from build123d import *

# Parameters (mm, degrees)
F1_DEPTH = 3.81
F2_R     = 8.89
F3_DEPTH = 2.54
F4_R     = 7.493
F5_DEPTH = 3.175
F6_R     = 0.4911819864


with BuildPart() as f1:
    # F0 (on Front) → F1 (new body)
    with BuildSketch(Plane.XZ):
        with BuildLine():
            ThreePointArc((8.8754738465, -0.508), (8.8863677196, -0.2541038219), (8.89, 0))
            ThreePointArc((8.89, 0), (7.6804215502, 4.4769660275), (4.3808380628, 7.7356549734))
            add(Edge.make_bspline(
                [(2.7757389763, 8.4455534535), (3.2888417453, 8.2703062234), (3.8159102337, 8.0198976132), (4.3808380628, 7.7356549734)],
                knots=[0.1783179795, 0.1783179795, 0.1783179795, 0.1783179795, 0.2655314771, 0.2655314771, 0.2655314771, 0.2655314771], degree=3))
            ThreePointArc((2.7757389763, 8.4455534535), (2.4438853282, 8.5474864435), (2.1083049646, 8.6363852494))
            add(Edge.make_bspline(
                [(0, 8.89), (0.577506035, 8.8570186599), (1.3119112895, 8.8227589155), (2.1083049646, 8.6363852494)],
                knots=[0, 0, 0, 0, 0.1399319156, 0.1399319156, 0.1399319156, 0.1399319156], degree=3))
            add(Edge.make_bspline(
                [(0, 8.89), (-0.577506035, 8.8570186599), (-1.3119112895, 8.8227589155), (-2.1083049646, 8.6363852494)],
                knots=[0, 0, 0, 0, 0.1399319156, 0.1399319156, 0.1399319156, 0.1399319156], degree=3))
            ThreePointArc((-2.1083049646, 8.6363852494), (-2.4438853282, 8.5474864435), (-2.7757389763, 8.4455534535))
            add(Edge.make_bspline(
                [(-2.7757389763, 8.4455534535), (-3.2888417453, 8.2703062234), (-3.8159102337, 8.0198976132), (-4.3808380628, 7.7356549734)],
                knots=[0.1783179795, 0.1783179795, 0.1783179795, 0.1783179795, 0.2655314771, 0.2655314771, 0.2655314771, 0.2655314771], degree=3))
            ThreePointArc((-4.3808380628, 7.7356549734), (-7.8052490793, 4.255606515), (-8.8754738465, -0.508))
            Line((-8.8754738465, -0.508), (-5.2194662387, -0.508))
            Line((-5.2194662387, -0.508), (-5.7473639175, 0.0198976788))
            Line((-5.7473639175, 0.0198976788), (0, 5.7672615963))
            Line((0, 5.7672615963), (5.7473639175, 0.0198976788))
            Line((5.7473639175, 0.0198976788), (5.2194662387, -0.508))
            Line((5.2194662387, -0.508), (8.8754738465, -0.508))
        make_face()
        with BuildLine():
            ThreePointArc((4.3808380628, 7.7356549734), (7.6804215502, 4.4769660275), (8.89, 0))
            ThreePointArc((8.89, 0), (8.8863677196, -0.2541038219), (8.8754738465, -0.508))
            Line((8.8754738465, -0.508), (20.32, -0.508))
            add(Edge.make_bspline(
                [(4.3808380628, 7.7356549734), (5.5525412949, 7.1461141461), (9.398567587, 5.0276978273), (19.2176653381, 4.6545545686), (20.0494547253, 0.2736910266), (20.32, -0.508)],
                knots=[0.2655314771, 0.2655314771, 0.2655314771, 0.2655314771, 0.4464188962, 0.7868227895, 1, 1, 1, 1], degree=3))
        make_face()
        with BuildLine():
            ThreePointArc((-8.8754738465, -0.508), (0, -8.89), (8.8754738465, -0.508))
            Line((8.8754738465, -0.508), (5.2194662387, -0.508))
            Line((5.2194662387, -0.508), (0, -5.7274662387))
            Line((0, -5.7274662387), (-5.2194662387, -0.508))
            Line((-5.2194662387, -0.508), (-8.8754738465, -0.508))
        make_face()
        with BuildLine():
            Line((-20.32, -0.508), (-8.8754738465, -0.508))
            ThreePointArc((-8.8754738465, -0.508), (-7.8052490793, 4.255606515), (-4.3808380628, 7.7356549734))
            add(Edge.make_bspline(
                [(-4.3808380628, 7.7356549734), (-5.5525412949, 7.1461141461), (-9.398567587, 5.0276978273), (-19.2176653381, 4.6545545686), (-20.0494547253, 0.2736910266), (-20.32, -0.508)],
                knots=[0.2655314771, 0.2655314771, 0.2655314771, 0.2655314771, 0.4464188962, 0.7868227895, 1, 1, 1, 1], degree=3))
        make_face()
    extrude(amount=F1_DEPTH)

    # F2 (on face) → F3 (join)
    with BuildSketch(Plane.XZ.offset(3.81)):
        Circle(F2_R)
        Polygon((-5.7473639175, 0.0198976788), (0, 5.7672615963), (5.7473639175, 0.0198976788), (0, -5.7274662387), align=None, mode=Mode.SUBTRACT)
    extrude(amount=F3_DEPTH)

    # F4 (on face) → F5 (join)
    with BuildSketch(Plane.XZ.offset(6.35)):
        Circle(F4_R)
        Polygon((0, -5.7274662387), (-5.7473639175, 0.0198976788), (0, 5.7672615963), (5.7473639175, 0.0198976788), align=None, mode=Mode.SUBTRACT)
    extrude(amount=F5_DEPTH)

    # F6
    f6_edges = [f1.edges().sort_by_distance(p)[0] for p in [
        (20.32, -1.905, -0.508),
        (-20.32, -1.905, -0.508),
    ]]
    fillet(f6_edges, radius=F6_R)


solid = f1.part
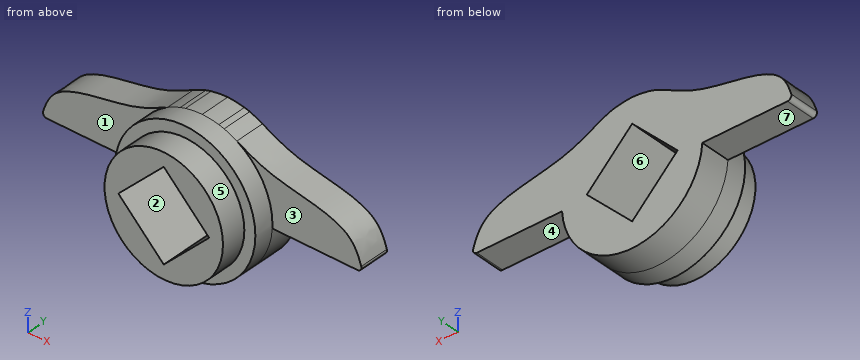
Could you check a few things on this model? Use its own coordinates, in mm. Face numbers are marked on the shaded views. A direction names the side the tool comes from. Round coordinates to 2 decimals unless told otherwise and drop trailing zeros. Write each loop counter-clockwise with the first axis right and the second up, starting at its lowest first coordinate (ties: lowest second). Pieces come first, ordered by that corner, then holes. Notation, with made-up numbers: (-28, 35.5) - (24, 35.5) arc R26 ccw to (24, 69.5) - close; hole circle Ø4 at (35, 80.25). An arc over 180 degrees is marked (long way). Put each result on its own line as item: value. Start each with the question number.
(1) Thinking about a two-plate mould opening in X: for the marked faces 5, 6 and 7, which applies, released by +X, released by -X, zero draft, split by the parting line, or undercut?
(2) I want a section at C-C, the plane z = -3.25. Please give me the cut outline in (x, y) (3 decimals), plus the area to 3 significant figures.
(3) I want a section at B-B, the plane z = -1. Please give me the cut outline in (x, y) (3 decimals), plus the area to 3 significant figures.
(4) I want a section at A-A, the plane y = -5.25. Please give me the cut outline in (x, z).
(5) Will these pins go through, and if not, where does the flat tip stop? pin 1 (1 mm diameter, centred on x = -15.5, z = 2.5, fed in from +Y); pin 2 (3 mm diameter, centred on y = -3, z = 4.5, fed in from -X); pin 3 (2 mm diameter, centred on y = -5.5, z = -3.5, fed in from +X); pin 4 (1.5 mm diameter, centred on x = -4.5, y = -7.5, fed in from +Z).
(6) I need wall thicknesses on probe 1 along Y at (x, z) = (18, 1); probe 2 along X at (y, z) = (-2.25, -0.25); probe 3 along X at (y, z) = (-6, 1). Which ranges of each line are inside material? Lowest first, please.
(7) For the marked faces 1, 2, 3 and 4, which set-ups out of +Z, -Z, +X, -X, +Y, -Y let a thin tool reach every point of the face, with its end or its side?
Here are the results:
1. face 5: split by the parting line
1. face 6: undercut
1. face 7: zero draft
2. outline: (-8.275, -6.35) - (-6.751, -6.35) - (-6.751, -9.525) - (-2.477, -9.525) - (-2.477, 0) - (-8.275, 0) - close; (2.477, -9.525) - (6.751, -9.525) - (6.751, -6.35) - (8.275, -6.35) - (8.275, 0) - (2.477, 0) - close
2. area: 101 mm^2
3. outline: (-8.834, -6.35) - (-7.426, -6.35) - (-7.426, -9.525) - (-4.727, -9.525) - (-4.727, 0) - (-8.834, 0) - close; (4.727, -9.525) - (7.426, -9.525) - (7.426, -6.35) - (8.834, -6.35) - (8.834, 0) - (4.727, 0) - close
3. area: 69.3 mm^2
4. outline: circle Ø17.78 at (0, 0); hole (-5.75, 0.02) - (0, -5.73) - (5.75, 0.02) - (0, 5.77) - close
5. pin 1: stops at y = 0
5. pin 2: stops at x = -18.48
5. pin 3: stops at x = 8.53
5. pin 4: stops at z = 6.49
6. probe 1: y = -3.81 to 0
6. probe 2: x = -20.09 to -5.48, 5.48 to 20.09
6. probe 3: x = -8.83 to -4.77, 4.77 to 8.83
7. face 1: +Z, -X, -Y
7. face 2: +Y, -Y
7. face 3: +Z, +X, -Y
7. face 4: -Z, +X, +Y, -Y
